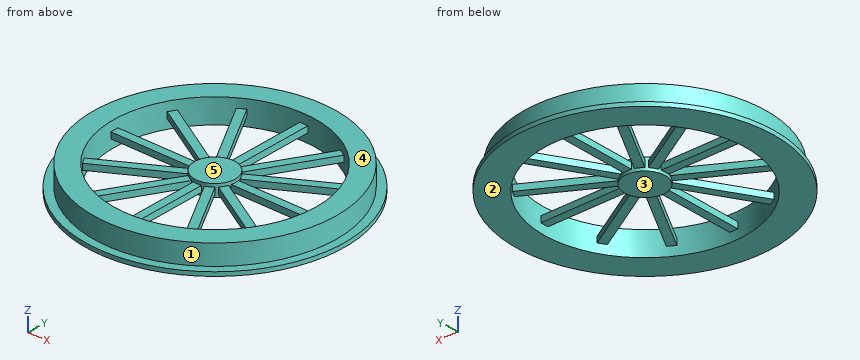
Autodesk Inventor part; units mm, degrees
ref_plane "YZ Plane" through (0, 0, 0) normal (1, 0, 0) x (0, 1, 0)
ref_plane "XZ Plane" through (0, 0, 0) normal (0, 1, 0) x (-1, 0, 0)
ref_plane "XY Plane" through (0, 0, 0) normal (0, 0, 1) x (1, 0, 0)
sketch "Sketch1" plane through (0, 0, 0) normal (0, 0, 1) x (1, 0, 0)
  circle A0 centre (0, 0) radius 127
  dimension "d0" = 254
extrude "Extrusion1" add sketch "Sketch1" along normal mid plane 76.2
sketch "Sketch2" plane through (0, 0, 0) normal (0, 0, 1) x (1, 0, 0)
  circle A0 centre (0, 0) radius 127 construction
  line L0 (-25.4, 124.4341) -> (25.4, 124.4341)
  line L1 (25.4, 124.4341) -> (25.4, 632.4341)
  line L2 (25.4, 632.4341) -> (-25.4, 632.4341)
  line L3 (-25.4, 632.4341) -> (-25.4, 124.4341)
  dimension "d3" = 50.8
  dimension "d4" = 508
extrude "Extrusion2" add sketch "Sketch2" along normal mid plane 38.1
pattern_circular "Circular Pattern1" count 12 over 360 about axis through (0, 0, -10) along (0, 0, 1) of "Extrusion2"
sketch "Sketch3" plane through (0, 0, 0) normal (0, 0, 1) x (1, 0, 0)
  circle A0 centre (0, 0) radius 632.4341
  line L0 (25.4, 632.4341) -> (-25.4, 632.4341)
  arc A1 (-95.0631, 84.2141) -> (-120.4631, 40.22) centre (0, 0) ccw
  circle A2 centre (0, 0) radius 759.4341
  point P0 (0, 632.4341)
  dimension "d10" = 127
extrude "Extrusion3" add sketch "Sketch3" along normal mid plane 152.4
sketch "Sketch5" plane through (0, 0, -76.2) normal (0, 0, -1) x (-1, 0, 0)
  circle A0 centre (0, 0) radius 810.2341
  circle A1 centre (0, 0) radius 759.4341
  circle A2 centre (0, 0) radius 759.4341
  dimension "d13" = 50.8
extrude "Extrusion4" add sketch "Sketch5" against normal blind 25.4
properties part number "wheel"
For this review, take the finished solid that the model builds, in its own axes (mm). Face numbers are marked on the shaded views. A direction names the side the tool comes from. Round coordinates to 2 decimals unless told otherwise and drop trailing zeros. Write each loop counter-clockwise with the first axis right and the second up, starting at its lowest first coordinate (ties: lowest second). Pieces come first, ordered by that corner, then holes. Notation, with made-up numbers: M 64,76.5 L 96,76.5 A28 cw 96,106.5 Z; hole C 72,63.5 d2. An arc over 180 degrees is marked long. Write item = value, one per line. Start each with the question number.
(1) The part is to be moulded in two halves that separate along X. For the marked faces 1, 2 and 3, say which applies: +X half, -X half, draft (parallel to the pull), parting line (faces both ways), or undercut.
(2) Clearance check with flat-ended pins moving along their axes: pin 1 Ø19 at (x, z) = (-419, -7) entering from -Y; pin 2 Ø19 at (y, z) = (-340, 3) entering from -X; pin 3 Ø4 at (y, z) = (342.5, -30.5) entering from -X. State where each tip first meets the part, or that it passes through.
(3) We need section A-A (x = 0). Give the boundary of the cut face in (y, z).
(4) For the marked faces 4 and 5, list the 3-axis set-ups (+Z, -Z, +X, -X, +Y, -Y) from which the entire face can be reached by the end or side of a thin tool; tool diameter is ignored.
(5) We need section B-B (y = 167.5). Give the number of separate pieces and of enclosed holes in the cut face, then the cut area to 3 significant figures.
(6) We need section D-D (x = 367). Give the boundary of the cut face in (y, z), then the cut area to 3 significant figures.
(7) For line 1 along X through (y, z) = (0, -37); line 2 along Y through (x, z) = (111, -14.5), list the stretches that pass through material, from the lowest coordinate up.
Results found:
q1.face_1 = parting line
q1.face_2 = draft
q1.face_3 = undercut
q2.pin_1 = -639.57
q2.pin_2 = -683.75
q2.pin_3 = -678.82
q3.outline = M -810.23,-76.2 L -632.43,-76.2 L -632.43,-19.05 L -127,-19.05 L -127,-38.1 L 127,-38.1 L 127,-19.05 L 632.43,-19.05 L 632.43,-76.2 L 810.23,-76.2 L 810.23,-50.8 L 759.43,-50.8 L 759.43,76.2 L 632.43,76.2 L 632.43,19.05 L 127,19.05 L 127,38.1 L -127,38.1 L -127,19.05 L -632.43,19.05 L -632.43,76.2 L -759.43,76.2 L -759.43,-50.8 L -810.23,-50.8 Z
q4.face_4 = +Z, +X, -X, +Y, -Y
q4.face_5 = +Z
q5.separate_pieces = 7
q5.enclosed_holes = 0
q5.area = 56,700 mm²
q6.outline = M -722.35,-76.2 L -515.06,-76.2 L -515.06,76.2 L -664.87,76.2 L -664.87,-50.8 L -722.35,-50.8 Z; M -241.22,-19.05 L -182.56,-19.05 L -182.56,19.05 L -241.22,19.05 Z; M -25.4,-19.05 L 25.4,-19.05 L 25.4,19.05 L -25.4,19.05 Z; M 182.56,-19.05 L 241.22,-19.05 L 241.22,19.05 L 182.56,19.05 Z; M 515.06,-76.2 L 722.35,-76.2 L 722.35,-50.8 L 664.87,-50.8 L 664.87,76.2 L 515.06,76.2 Z
q6.area = 55,000 mm²
q7.line_1 = -759.43 to -632.43, -127 to 127, 632.43 to 759.43
q7.line_2 = -751.28 to -622.62, -243.06 to -141.46, -93.42 to 93.42, 141.46 to 243.06, 622.62 to 751.28
